Design review of the part built by this model. Coordinates are the model's own, in mm. Face numbers are marked on the shaded views. A direction names the side the tool comes from. Coordinates: 2 decimals unless noted, no trailing zeros. Write each loop counter-clockwise with the first axis right and the second up, starting at its lowest first coordinate (ties: lowest second). Pieces come first, ordered by that corner, then holes. Notation, with made-up numbers: (62, 69.5) - (96, 69.5) arc R15 ccw to (96, 75.5) - close; hole circle Ø9 at (9.25, -2.75). An arc over 180 degrees is marked (long way). Answer as a JSON object with one key per item and string values.
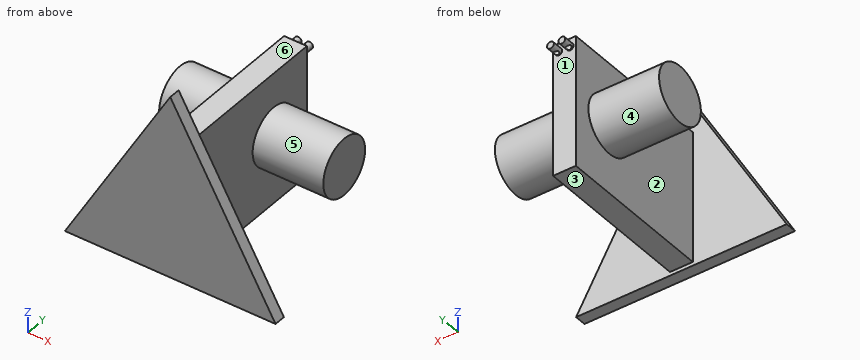
```python
from build123d import *

# Parameters (mm, degrees)
BOSS_EXTRUDE1_DEPTH    = 10
SKETCH6_W              = 20
SKETCH6_H              = 64.955790415
SKETCH6_H_2            = 50.098640903
BOSS_EXTRUDE4_DEPTH    = 140
SKETCH7_R              = 25
BOSS_EXTRUDE5_DEPTH    = 62
SKETCH12_R             = 3
BOSS_EXTRUDE6_DEPTH    = 10
CUT_EXTRUDE1_START     = 54.455790306
CUT_EXTRUDE1_OUTLINE_R = 2.25
CUT_EXTRUDE1_DEPTH     = 6.544209694


with BuildPart() as part:
    # Sketch1 → Boss-Extrude1 (new body)
    with BuildSketch(Plane(origin=(0, 0, 0), x_dir=(1, 0, 0), z_dir=(0, 1, 0))):
        Polygon((0, -106.666666667), (92.37604307, 53.333333333), (-92.37604307, 53.333333333), align=None)
    extrude(amount=BOSS_EXTRUDE1_DEPTH)

    # Sketch6 → Boss-Extrude4 (add)
    with BuildSketch(Plane(origin=(0, 10, 0), x_dir=(1, 0, 0), z_dir=(0, 1, 0))):
        with Locations((0, -32.477895208)):
            Rectangle(SKETCH6_W, SKETCH6_H)
        with Locations((0, 25.049320452)):
            Rectangle(SKETCH6_W, SKETCH6_H_2)
    extrude(amount=BOSS_EXTRUDE4_DEPTH)

    # Sketch7 → Boss-Extrude5 (add)
    with BuildSketch(Plane(origin=(10, 0, 0), x_dir=(0, 0, -1), z_dir=(1, 0, 0))):
        with Locations((-9.955790415, 110)):
            Circle(SKETCH7_R)
    boss_extrude5 = extrude(amount=BOSS_EXTRUDE5_DEPTH)

    # Mirror1: Boss-Extrude5 across plane
    add(boss_extrude5.mirror(Plane(origin=(0, 0, 0), x_dir=(0, 0, 1), z_dir=(1, 0, 0))))

    # Sketch12 → Boss-Extrude6 (add)
    with BuildSketch(Plane(origin=(0, 150, 0), x_dir=(1, 0, 0), z_dir=(0, 1, 0))):
        with Locations(Location((5, -57.455790415, 0), (0, 0, 270))):
            Circle(SKETCH12_R)
        with Locations(Location((-5, -57.455790415, 0), (0, 0, 270))):
            Circle(SKETCH12_R)
    extrude(amount=BOSS_EXTRUDE6_DEPTH)

    # Cut-Extrude1: read off the stored shape, not the designer's step
    # Cut-Extrude1 outline → Cut-Extrude1 (cut)
    with BuildSketch(Plane.XY.offset(CUT_EXTRUDE1_START)):
        with Locations((-5.5, 152.935681358)):
            Circle(CUT_EXTRUDE1_OUTLINE_R)
        with Locations((5.176294741, 152.935681358)):
            Circle(CUT_EXTRUDE1_OUTLINE_R)
    extrude(amount=CUT_EXTRUDE1_DEPTH, mode=Mode.SUBTRACT)


solid = part.part
```
(1) For pin 1 (6 mm diameter, centred on x = -71, y = 117, fed in from -Z); pin 2 (2 mm diameter, centred on y = 51, z = -28.5, fed in from +X); pin 3 (22 mm diameter, centred on x = 2.5, y = 81, fed in from +Z), all flat-tipped, find the tip position at first contact; note any pin that passes through.
Solved:
{"pin 1": "stops at z = -14.72", "pin 2": "stops at x = 10", "pin 3": "stops at z = 64.96"}
(2) Take a section at C-C, the plane x = 14.5. Write out the cut boundary in (y, z), and give its area (3 significant figures).
Solved:
{"outline": "(0, -53.33) - (10, -53.33) - (10, 81.55) - (0, 81.55) - close; circle Ø50 at (110, 9.96)", "area": "3,310 mm^2"}
(3) To check wall thickness, follow line 1 (Y direction, x = -45.5, z = 11); line 2 (Y direction, x = -5.5, z = 59.25); line 3 (X direction, y = 131.5, z = 59.5). State the ranges of each line that lie inside material, in increasing order. Write a range as from..to.
Solved:
{"line 1": "y = 0..10, 85.02..134.98", "line 2": "y = 0..150.69, 155.19..160", "line 3": "x = -10..10"}
(4) The part is to be moulded in two halves that separate along Y. For the marked faces 1, 2 and 3, say which applies: pulls with the +Y half, pulls with the -Y half, needs draft (parallel to the pull), parting line crosses it, or undercut.
Solved:
{"face 1": "pulls with the +Y half", "face 2": "undercut", "face 3": "needs draft"}
(5) Tool access review of the marked faces 4, 5 and 6: name each direction out of +Z, -Z, +X, -X, +Y, -Y from which nothing blocks a thin tool from reaching the whole face with its end or side.
Solved:
{"face 4": "-X", "face 5": "+X", "face 6": "+Z, +X, -X, +Y"}
(6) Take a section at D-D, the plane x = 59. Write out the cut boundary in (y, z), and give its area (3 significant figures).
Solved:
{"outline": "(0, -53.33) - (10, -53.33) - (10, 4.48) - (0, 4.48) - close; circle Ø50 at (110, 9.96)", "area": "2,540 mm^2"}
(7) Take a section at B-B, the plane z = 29. Write out the cut boundary in (x, y), and give its area (3 significant figures).
Solved:
{"outline": "(-72, 93.8) - (-10, 93.8) - (-10, 10) - (-44.84, 10) - (-44.84, 0) - (44.84, 0) - (44.84, 10) - (10, 10) - (10, 93.8) - (72, 93.8) - (72, 126.2) - (10, 126.2) - (10, 150) - (-10, 150) - (-10, 126.2) - (-72, 126.2) - close", "area": "7,710 mm^2"}
(8) Take a section at A-A, the plane y = 126. Write out the cut boundary in (x, z), and give its area (4 significant figures).
Solved:
{"outline": "(-72, -9.25) - (-10, -9.25) - (-10, -50.1) - (10, -50.1) - (10, -9.25) - (72, -9.25) - (72, 29.17) - (10, 29.17) - (10, 64.96) - (-10, 64.96) - (-10, 29.17) - (-72, 29.17) - close", "area": "7,065 mm^2"}
